from build123d import *

# Parameters (mm, degrees)
SKETCH1_R      = 1.2295
BASENUT_DEPTH  = 1.72
EXTRUDE1_START = 2.78
SKETCH2_R      = 2.66
SKETCH2_R_2    = 1.2295
EXTRUDE1_DEPTH = 2.78
CHAMFER1_SIZE  = 0.1064


with BuildPart() as part:
    # Sketch1 → BaseNut (new body)
    with BuildSketch(Plane.XY):
        Polygon((1.58771324, -2.75), (3.175426481, 0), (1.58771324, 2.75), (-1.58771324, 2.75), (-3.175426481, 0), (-1.58771324, -2.75), align=None)
        Circle(SKETCH1_R, mode=Mode.SUBTRACT)
    extrude(amount=-BASENUT_DEPTH)

    # Sketch3 → Double-Chamfer (revolve, cut)
    with BuildSketch(Plane(origin=(0, 0, 0), x_dir=(1, 0, 0), z_dir=(0, 1, 0))):
        Polygon((2.285, 1.72), (3.175426481, 1.72), (3.175426481, 1.205912032), align=None)
        Polygon((3.175426481, 0.514087968), (2.285, 0), (3.175426481, 0), align=None)
    revolve(axis=Axis((0, 0, -16.31077227), (0, 0, 1)), mode=Mode.SUBTRACT)

    # Sketch2 → Extrude1 (add)
    with BuildSketch(Plane(origin=(20.087129569, -4.281493882, 0), x_dir=(1, 0, 0), z_dir=(0, 0, 1)).offset(EXTRUDE1_START)):
        with Locations(Location((-20.087129569, 4.281493882, 0), (0, 0, 180))):
            Circle(SKETCH2_R)
        with Locations((-20.087129569, 4.281493882)):
            Circle(SKETCH2_R_2, mode=Mode.SUBTRACT)
    extrude(amount=-EXTRUDE1_DEPTH)

    # Sketch5 → EndChamfer (revolve, cut)
    with BuildSketch(Plane(origin=(0, 0, 0), x_dir=(1, 0, 0), z_dir=(0, 1, 0))):
        Polygon((1.2295, 1.72), (1.725, 1.72), (1.2295, 1.2245), align=None)
    revolve(axis=Axis((0, 0, -16.800797033), (0, 0, 1)), mode=Mode.SUBTRACT)

    # Chamfer1
    chamfer1_edges = [part.edges().sort_by_distance(p)[0] for p in [
        (2.66, 0, 2.78),
    ]]
    chamfer(chamfer1_edges, length=CHAMFER1_SIZE)


solid = part.part
Check sheet for the modelled part. Datum: model origin and axes. Units: mm. Round coordinates to 2 decimals unless told otherwise and drop trailing zeros. Order: outer loops, then holes, each group sorted by start corner. A loop starts at its lowest first (then second) coordinate and runs counter-clockwise, first axis right, second up. Notation, with made-up numbers: M 52.25,-19 L 87.25,-19 A22 cw 87.25,14 Z; hole C 29,70.25 d10. An arc over 180 degrees is marked long. One line per item, written item: value. Start each with the question number.
1. Scan lines: line 1 along Y through (x, z) = (0, 0.8); line 2 along Y through (x, z) = (-0.5, -0.6); line 3 along Y through (x, z) = (-2, 2.35). Record each from-to range of solid material in increasing order.
2. Gauge pin test, flat ends, axial feed: P1, Ø3, axis at x = 2, y = 2, coming from the +Z side; P2, Ø2, axis at x = -1.5, z = 1, coming from the +Y side; P3, Ø2, axis at x = -0.5, z = 1.5, coming from the +Y side; P4, Ø3, axis at x = 0, y = 0, coming from the -Z side (3 decimals). Record the tip position at first contact, or that the pin passes through.
3. Section check C-C on z = -0.1. Enter the section's corners in (x, y).
4. Section check B-B on z = 1.35. Enter the section's corners in (x, y).
5. Release check for a two-part mould opening along Y. For faces 1 (the flat face through (2.39, 1.36, -0.85)), 2 (the cylindrical face through (-2.537, -0.799, 1.356)), 3 (the cylindrical face through (-0.976, -0.748, 0.806)) record: released by +Y, released by -Y, zero draft, split by the parting line, or undercut.
Results found:
1. line 1: -2.66 to -1.23, 1.23 to 2.66
1. line 2: -2.75 to -1.12, 1.12 to 2.75
1. line 3: -1.75 to 1.75
2. P1: z = 2.78
2. P2: y = 2.61
2. P3: y = 2.66
2. P4: z = -1.495
3. outline: C 0,0 d4.92; hole C 0,0 d2.46
4. outline: C 0,0 d5.32; hole C 0,0 d2.46
5. face 1: released by +Y
5. face 2: split by the parting line
5. face 3: undercut
